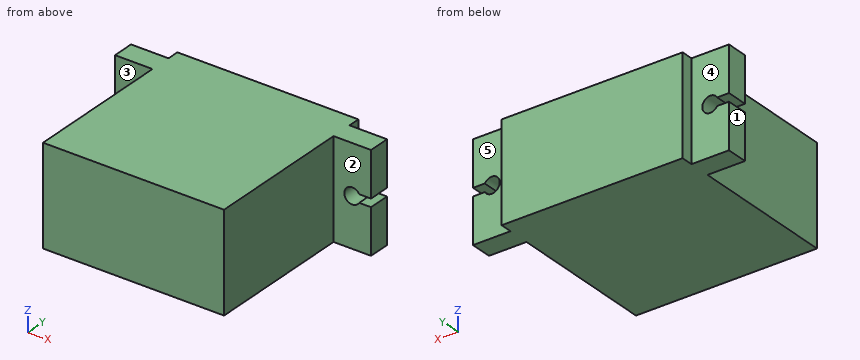
from build123d import *

# Parameters (mm, degrees)
EXTRUSION2_CUT_DEPTH = 12.3
EXTRUSION1_DEPTH     = 12.3


with BuildPart() as extrusion2_cut:
    with BuildSketch(Plane(origin=(22.7, -1.5, 0), x_dir=(1, 0, 0), z_dir=(0, 1, 0))):
        with BuildLine():
            Line((-25.916025, 6.65), (-27.4, 6.65))
            Line((-27.4, 6.65), (-27.4, 5.65))
            Line((-27.4, 5.65), (-25.916025, 5.65))
            ThreePointArc((-25.916025, 5.65), (-24.05, 6.15), (-25.916025, 6.65))
        make_face()
        with BuildLine():
            Line((3.216025, 5.65), (4.7, 5.65))
            Line((4.7, 5.65), (4.7, 6.65))
            Line((4.7, 6.65), (3.216025, 6.65))
            ThreePointArc((3.216025, 6.65), (1.35, 6.15), (3.216025, 5.65))
        make_face()
    extrude(amount=-EXTRUSION2_CUT_DEPTH)


with BuildPart() as extrusion2:
    with BuildSketch(Plane.XY):
        Polygon((22.7, -22.7), (22.7, -4.2), (27.4, -4.2), (27.4, -1.5), (22.7, -1.5), (22.7, 0), (0, 0), (0, -1.5), (-4.7, -1.5), (-4.7, -4.2), (0, -4.2), (0, -22.7), align=None)
    extrude(amount=-EXTRUSION1_DEPTH)

    # Extrusion2: cut Extrusion2_Cut
    add(extrusion2_cut.part, mode=Mode.SUBTRACT)


solid = extrusion2.part
The listing builds one solid part. Answer for the finished solid, in the listing's coordinates (mm). Face numbers are marked on the shaded views. A direction names the side the tool comes from. Give positions to 0.01 mm unless a question says otherwise; leave off trailing zeros. Loops run counter-clockwise (first coordinate to the right, second up) from the corner with the lowest first, then second, coordinate; pieces in that order, holes last. Notation, with made-up numbers: (-19, -34) - (11, -34) arc R21 ccw to (11, -28) - close; hole circle Ø6 at (-27, 63.5). An arc over 180 degrees is marked (long way). Use one line per item in the form item = value.
1. Section D-D on y = -8 is taken. Give the vertices of the cut face in (x, z).
Calculated:
outline = (0, -12.3) - (22.7, -12.3) - (22.7, 0) - (0, 0) - close
2. Which of the six approach directions +Z, -Z, +X, -X, +Y, -Y give full straight-line access (tool end or side, diameter ignored) to the marked faces 1, 2, 3, 4 and 5?
Calculated:
face_1 = +Z, -Z, -X, +Y, -Y
face_2 = +Z, -Z, +X, -Y
face_3 = +Z, -Z, -X, -Y
face_4 = +Z, -Z, -X, +Y
face_5 = +Z, -Z, +X, +Y
3. Section B-B on z = -8.75 is taken. Give the vertices of the cut face in (x, y), then the cut area to 3 significant figures.
Calculated:
outline = (-4.7, -4.2) - (0, -4.2) - (0, -22.7) - (22.7, -22.7) - (22.7, -4.2) - (27.4, -4.2) - (27.4, -1.5) - (22.7, -1.5) - (22.7, 0) - (0, 0) - (0, -1.5) - (-4.7, -1.5) - close
area = 541 mm^2
4. Given pin 1 Ø0.8 at (y, z) = (-0.5, -6.5) entering from -X; pin 2 Ø0.7 at (x, y) = (-3.5, -2.5) entering from +Z; pin 3 Ø2.5 at (x, z) = (-1.5, -5) entering from -Y; pin 4 Ø5 at (x, z) = (-3, -3.5) entering from +Y, each flat-ended and moving along its own axis, determine where each tip first touches the part or whether it passes through.
Calculated:
pin_1 = 0
pin_2 = 0
pin_3 = -4.2
pin_4 = -1.5
5. Find the intervals of material crossed by line 1 along Z through (x, y) = (25.05, -3.6); line 2 along X through (y, z) = (-2.6, -6.15); line 3 along X through (y, z) = (-13.5, -4.75), in increasing order. Write a range as [from, to].
Calculated:
line_1 = [-12.3, -7.15], [-5.15, 0]
line_2 = [-1.35, 24.05]
line_3 = [0, 22.7]
6. Section A-A on x = -2.35 is taken. Give the vertices of the cut face in (y, z), then the cut area to 3 significant figures.
Calculated:
outline = (-4.2, -12.3) - (-1.5, -12.3) - (-1.5, -7.15) - (-4.2, -7.15) - close; (-4.2, -5.15) - (-1.5, -5.15) - (-1.5, 0) - (-4.2, 0) - close
area = 27.8 mm^2
